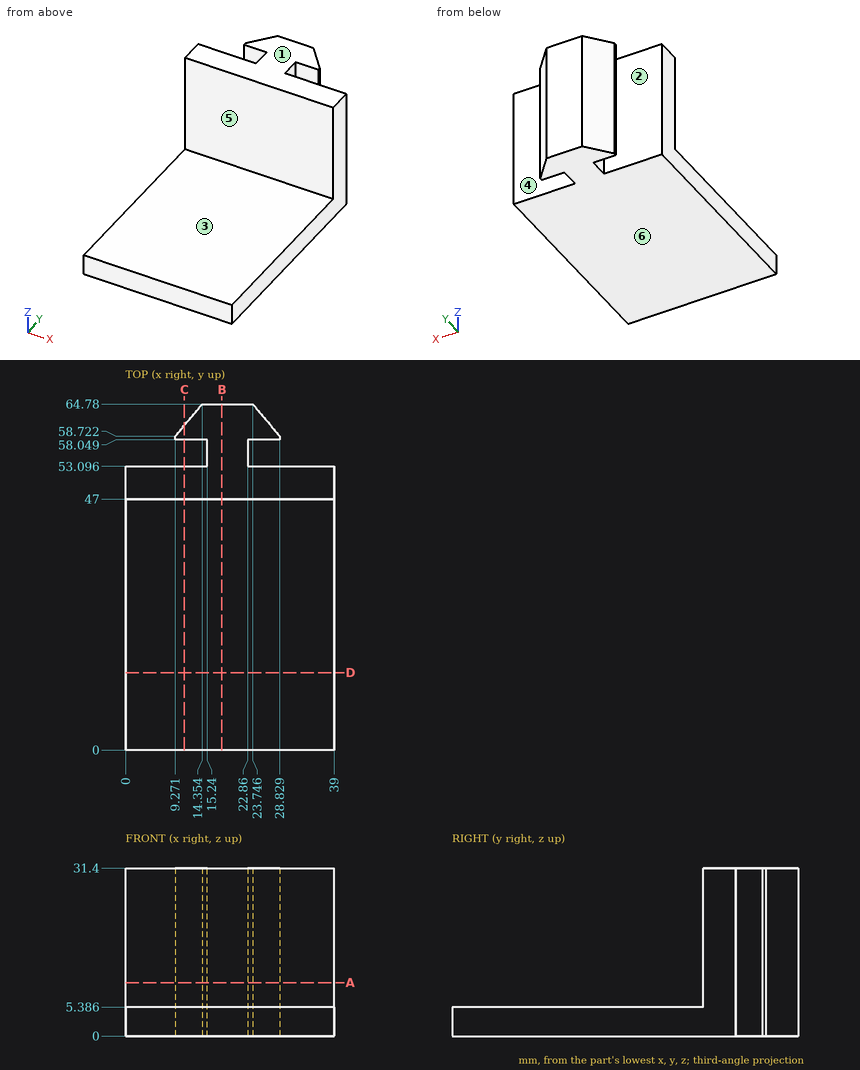
For this review, use the dimensioned drawing (mm, ordinates from the lowest corner) and the shaded views. A direction names the side the tool comes from. Give positions to 0.01 mm unless a question says otherwise; leave off trailing zeros. Write each loop counter-clockwise with the first axis right and the second up, starting at its lowest first coordinate (ties: lowest second). Pieces come first, ordered by that corner, then holes. Notation, with made-up numbers: M 32.25,-3.5 L 38.25,-3.5 A17 cw 38.25,24.5 Z; hole C -2.75,83.5 d10. An arc over 180 degrees is marked long. Answer as a JSON object with one key per item and string values. Group by question number.
1) Tool access review of the marked faces 1, 2 and 3: name each direction out of +Z, -Z, +X, -X, +Y, -Y from which nothing blocks a thin tool from reaching the whole face with its end or side.
2) For line 1 along Z through (x, y) = (22.5, 44); line 2 along Y through (x, z) = (22, 22.5); line 3 along Y through (x, z) = (4, 13.5), list the stretches that pass through material, from the lowest coordinate up.
3) Mouldability with a two-part tool opening along Y and no side actions: class the marked faces 4, 5 and 6 as released by +Y, released by -Y, zero draft, split by the parting line, or undercut.
4) We need section C-C (x = 11). Give the boundary of the cut face in (y, z), and give its area (3 significant figures).
5) We need section B-B (x = 18). Give the boundary of the cut face in (y, z).
6) We need section A-A (z = 10). Give the boundary of the cut face in (x, y), and give its area (3 significant figures).
7) Clearance check with flat-ended pins moving along their axes: pin 1 Ø8 at (x, z) = (21, 17.5) entering from -Y; pin 2 Ø1.5 at (y, z) = (56.5, 23.5) entering from +X; pin 3 Ø10 at (x, y) = (14, 11.5) entering from +Z. State where each tip first meets the part, or that it passes through.
8) We need section D-D (y = 14.5). Give the boundary of the cut face in (x, z).
Answer key:
{
 "1": {"face 1": "+Z, +X, -X, +Y, -Y", "face 2": "+Z, -Z, -X", "face 3": "+Z, +X, -X, -Y"},
 "2": {"line 1": "z = 0 to 5.39", "line 2": "y = 47 to 64.78", "line 3": "y = 47 to 53.1"},
 "3": {"face 4": "undercut", "face 5": "released by -Y", "face 6": "zero draft"},
 "4": {"outline": "M 0,0 L 53.1,0 L 53.1,31.4 L 47,31.4 L 47,5.39 L 0,5.39 Z; M 58.05,0 L 60.78,0 L 60.78,31.4 L 58.05,31.4 Z", "area": "530 mm²"},
 "5": {"outline": "M 0,0 L 64.78,0 L 64.78,31.4 L 47,31.4 L 47,5.39 L 0,5.39 Z"},
 "6": {"outline": "M 0,47 L 39,47 L 39,53.1 L 22.86,53.1 L 22.86,58.05 L 28.83,58.05 L 28.83,58.72 L 23.75,64.78 L 14.35,64.78 L 9.27,58.72 L 9.27,58.05 L 15.24,58.05 L 15.24,53.1 L 0,53.1 Z", "area": "376 mm²"},
 "7": {"pin 1": "stops at y = 47", "pin 2": "stops at x = 22.86", "pin 3": "stops at z = 5.39"},
 "8": {"outline": "M 0,0 L 39,0 L 39,5.39 L 0,5.39 Z"}
}
